```python
from build123d import *

# Parameters (mm, degrees)
Y_KSEKLIK_EKSTR_ZYON1_DEPTH = 20
IZIM6_R                     = 1.7
KES_EKSTR_ZYON2_DEPTH       = 20
KES_EKSTR_ZYON3_DEPTH       = 46
Y_KSEKLIK_EKSTR_ZYON2_DEPTH = 20
IZIM9_R                     = 1.7
IZIM9_R_2                   = 1.75
KES_EKSTR_ZYON4_DEPTH       = 46


with BuildPart() as part:
    # Çizim1 → Yükseklik-Ekstrüzyon1 (new body)
    with BuildSketch(Plane.XY):
        with BuildLine():
            Line((-3.5, 11.687172455), (-3.5, 20.580454312))
            Line((-3.5, 20.580454312), (-3.5, 24.580454312))
            Line((-3.5, 24.580454312), (-7, 24.580454312))
            Line((-7, 24.580454312), (-7, 20.580454312))
            Line((-7, 20.580454312), (-7, 14.053113534))
            ThreePointArc((-7, 14.053113534), (-15.647613909, 1.281475299), (-9.19317791, -12.726958785))
            Line((-9.19317791, -12.726958785), (-15.7, -43))
            Line((-15.7, -43), (15.7, -43))
            Line((15.7, -43), (9.881801455, -12.2))
            ThreePointArc((9.881801455, -12.2), (15.606258285, 1.713097297), (7, 14.053113534))
            Line((7, 14.053113534), (7, 20.580454312))
            Line((7, 20.580454312), (7, 24.580454312))
            Line((7, 24.580454312), (3.5, 24.580454312))
            Line((3.5, 24.580454312), (3.5, 20.580454312))
            Line((3.5, 20.580454312), (3.5, 11.687172455))
            ThreePointArc((3.5, 11.687172455), (0, -12.2), (-3.5, 11.687172455))
        make_face()
    extrude(amount=Y_KSEKLIK_EKSTR_ZYON1_DEPTH)

    # Çizim6 → Kes-Ekstrüzyon2 (cut)
    with BuildSketch(Plane(origin=(7, 0, 0), x_dir=(0, 0, -1), z_dir=(1, 0, 0))):
        with Locations((-10, 19.316783923)):
            Circle(IZIM6_R)
    extrude(amount=-KES_EKSTR_ZYON2_DEPTH, mode=Mode.SUBTRACT)

    # Çizim7 → Kes-Ekstrüzyon3 (cut)
    with BuildSketch(Plane.XY.offset(20)):
        Polygon((-15.7, -43), (-15.7, -19), (23.821750054, -19), (23.821750054, -48.375532492), (-15.7, -48.375532492), align=None)
    extrude(amount=-KES_EKSTR_ZYON3_DEPTH, mode=Mode.SUBTRACT)

    # Çizim8 → Yükseklik-Ekstrüzyon2 (add)
    with BuildSketch(Plane.XY.offset(20)):
        Polygon((-10.541491839, -19), (-25.541491839, -19), (-25.541491839, -24), (11.166338796, -24), (26.166338796, -24), (26.166338796, -19), (11.166338796, -19), align=None)
    extrude(amount=-Y_KSEKLIK_EKSTR_ZYON2_DEPTH)

    # Çizim9 → Kes-Ekstrüzyon4 (cut)
    with BuildSketch(Plane(origin=(0, -19, 0), x_dir=(1, 0, 0), z_dir=(0, 1, 0))):
        with Locations(Location((-20.541491839, -10, 0), (0, 0, 270))):
            Circle(IZIM9_R)
        with Locations(Location((21.166338796, -10, 0), (0, 0, 270))):
            Circle(IZIM9_R_2)
    extrude(amount=-KES_EKSTR_ZYON4_DEPTH, mode=Mode.SUBTRACT)


solid = part.part
```
Input: part model. Units: mm. Frame: model coordinates. A direction names the side the tool comes from. Give positions to 0.01 mm unless a question says otherwise; leave off trailing zeros. Write each loop counter-clockwise with the first axis right and the second up, starting at its lowest first coordinate (ties: lowest second). Pieces come first, ordered by that corner, then holes. Notation, with made-up numbers: (23, -26.75) - (36, -26.75) arc R18 ccw to (36, 8.25) - close; hole circle Ø4 at (65.5, 23). An arc over 180 degrees is marked (long way). Write item = value, one per line. Start each with the question number.
1. Section query B-B, the plane y = 0. Output: boundary loops of the cut face in (x, z), then the cut area to 3 significant figures.
2. Mould query, pull axis Y, two halves, no side actions, for faces 5 (the cylindrical face through (22.9, -21.46, 9.77)), 6 (the flat face through (5, 24.58, 10)), 7 (the cylindrical face through (-15.628, 1.506, 9.86)), 8 (the flat face through (19, -19, 10)). Classes: released by +Y, released by -Y, zero draft, split by the parting line, or undercut.
3. Section query A-A, the plane z = 10. Count the separate pieces of the cut face and the enclosed holes in it, then the cut area to 3 significant figures.
4. First-contact query: pin 1 Ø5 at (x, z) = (1.5, 8.5) entering from +Y; pin 2 Ø1.5 at (y, z) = (-5, 14.5) entering from -X; pin 3 Ø6.5 at (y, z) = (18.5, 9) entering from +X; pin 4 Ø5 at (x, z) = (0, 14) entering from +Y. Flat tips, straight axial feed; report the tip coordinate or a pass-through.
5. Section query D-D, the plane z = 12.75. Output: boundary loops of the cut face in (x, y), then the cut area to 3 significant figures.
6. Access query for faces 1 (the flat face through (-3.5, 17, 10)), 2 (the flat face through (-7, 19, 8)), 3 (the flat face through (10.533, -15.648, 9.86)), 4 (the flat face through (-9.86, -15.82, 9.86)). Directions: +Z, -Z, +X, -X, +Y, -Y. A direction counts if a zero-diameter tool reaches every point of the face in a straight line with its end or side. Return the directions, or none.
7. Ray query, L1, parallel to X at y = -21.35, z = 10; L2, parallel to X at y = 0.5, z = 10; L3, parallel to Y at x = 4, z = 11. Return the intervals inside material, ascending.
8. Section query C-C, the plane x = 13. Output: boundary loops of the cut face in (y, z).
Check sheet entries:
q1.outline = (-15.7, 0) - (-12.2, 0) - (-12.2, 20) - (-15.7, 20) - close; (12.2, 0) - (15.7, 0) - (15.7, 20) - (12.2, 20) - close
q1.area = 140 mm2
q2.face_5 = zero draft
q2.face_6 = released by +Y
q2.face_7 = undercut
q2.face_8 = undercut
q3.separate_pieces = 5
q3.enclosed_holes = 0
q3.area = 642 mm2
q4.pin_1 = 24.58
q4.pin_2 = -15.11
q4.pin_3 = 7
q4.pin_4 = -11.94
q5.outline = (-25.54, -24) - (26.17, -24) - (26.17, -19) - (11.17, -19) - (9.88, -12.2) arc R15.7 ccw to (7, 14.05) - (7, 24.58) - (3.5, 24.58) - (3.5, 11.69) arc R12.2 cw (long way) to (-3.5, 11.69) - (-3.5, 24.58) - (-7, 24.58) - (-7, 14.05) arc R15.7 ccw to (-9.19, -12.73) - (-10.54, -19) - (-25.54, -19) - close
q5.area = 701 mm2
q6.face_1 = +Z, -Z, +Y
q6.face_2 = +Z, -Z, -X, +Y
q6.face_3 = +Z, -Z, +X
q6.face_4 = +Z, -Z, -X
q7.L1 = -25.54 to -22.24, -18.84 to 19.42, 22.92 to 26.17
q7.L2 = -15.69 to -12.19, 12.19 to 15.69
q7.L3 = -24 to -11.53, 11.53 to 17.94, 20.69 to 24.58
q8.outline = (-24, 0) - (-19, 0) - (-19, 20) - (-24, 20) - close; (-8.8, 0) - (8.8, 0) - (8.8, 20) - (-8.8, 20) - close
